Part print with two shaded views. Sizes in mm from the minimum x, y, z corner. A direction names the side the tool comes from. Give positions to 0.01 mm unless a question says otherwise; leave off trailing zeros. Write each loop counter-clockwise with the first axis right and the second up, starting at its lowest first coordinate (ties: lowest second). Pieces come first, ordered by that corner, then holes. Notation, with made-up numbers: M -9,-32 L 46,-32 A23 ccw 46,-4 Z; hole C 77,78 d4. An arc over 180 degrees is marked long. Return JSON: item names as keys, results as strings. Group by question number.
Q1. Band-saw the part on D-D, the plane x = 31. Give the cut face in (y, z), then the cut area to 3 significant figures.
Q2. Band-saw the part on A-A, the plane z = 32.5. Give the cut face in (x, y), then the cut area to 3 significant figures.
Q3. Flat gauge pins, fed straight in: pin 1 Ø1.5 at (y, z) = (12.5, 15.5) entering from -X; pin 2 Ø16 at (x, y) = (23.5, 17.5) entering from +Z; pin 3 Ø3 at (y, z) = (36, 11) entering from +X; pin 4 Ø10 at (y, z) = (24.5, 26.5) entering from +X. Where does each tip first touch, or does it go through?
Q4. Wall check: probe 1 along Y at (x, z) = (15.5, 34); probe 2 along Z at (x, y) = (9, 9.5); probe 3 along X at (y, z) = (5.5, 21). Give the ranges that are in metal, low to high.
Q5. Band-saw the part on B-B, the plane y = 33. Give the cut face in (x, z).
Q6. Band-saw the part on C-C, the plane z = 8. Give the cut face in (x, y).
Q7. Tool access for the marked faces 1, 2, 3, 4 and 5: list every direction of +Z, -Z, +X, -X, +Y, -Y with a clear straight run to the whole face (end or side of a thin tool).
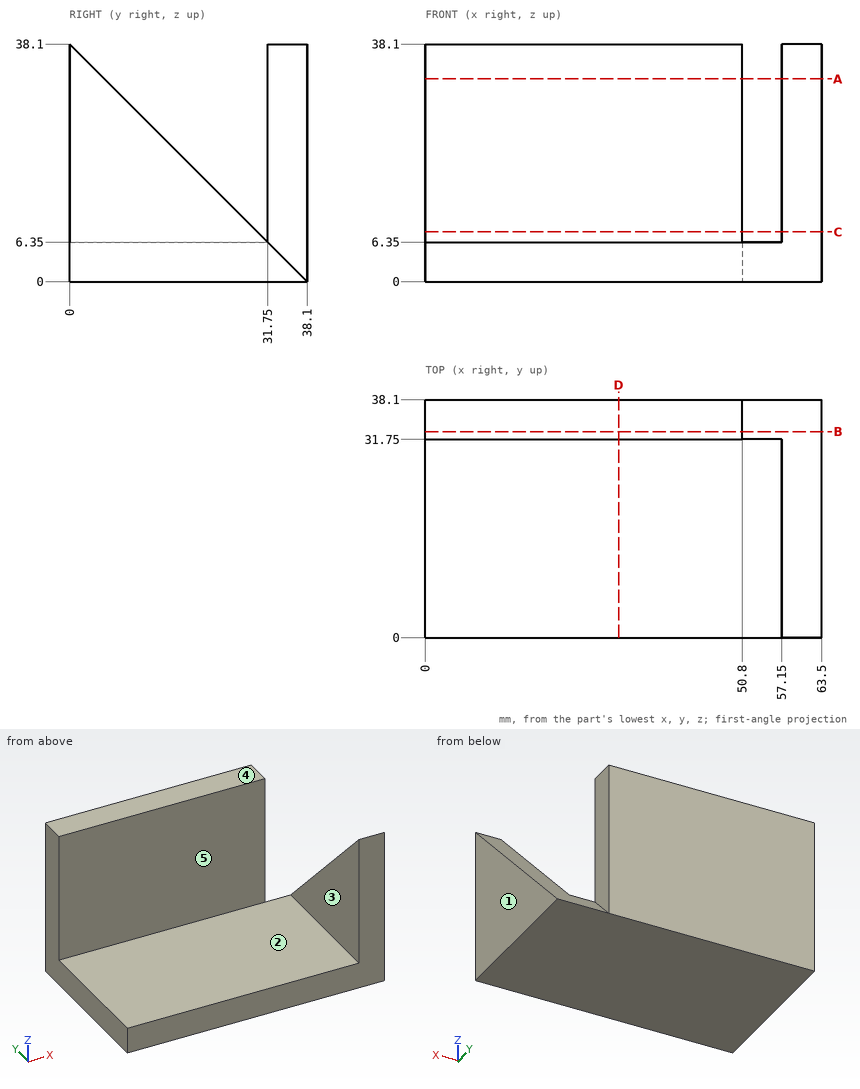
From the geometry:
{
 "1": {"outline": "M 0,0 L 38.1,0 L 38.1,38.1 L 31.75,38.1 L 31.75,6.35 L 0,6.35 Z", "area": "444 mm^2"},
 "2": {"outline": "M 0,31.75 L 50.8,31.75 L 50.8,38.1 L 0,38.1 Z; M 57.15,0 L 63.5,0 L 63.5,5.6 L 57.15,5.6 Z", "area": "358 mm^2"},
 "3": {"pin 1": "stops at x = 57.15", "pin 2": "stops at z = 6.35", "pin 3": "stops at x = 50.8", "pin 4": "passes through"},
 "4": {"probe 1": "y = 31.75 to 38.1", "probe 2": "z = 0 to 6.35", "probe 3": "x = 57.15 to 63.5"},
 "5": {"outline": "M 0,0 L 63.5,0 L 63.5,5.1 L 50.8,5.1 L 50.8,38.1 L 0,38.1 Z"},
 "6": {"outline": "M 0,31.75 L 50.8,31.75 L 50.8,38.1 L 0,38.1 Z; M 57.15,0 L 63.5,0 L 63.5,30.1 L 57.15,30.1 Z"},
 "7": {"face 1": "+Z, -Z, +X, +Y, -Y", "face 2": "+Z, -X, -Y", "face 3": "+Z, -X, +Y, -Y", "face 4": "+Z, +X, -X, +Y, -Y", "face 5": "+Z, +X, -X, -Y"}
}
